Design review of the part built by this model. Coordinates are the model's own, in mm. Face numbers are marked on the shaded views. A direction names the side the tool comes from. Give positions to 0.01 mm unless a question says otherwise; leave off trailing zeros. Loops run counter-clockwise (first coordinate to the right, second up) from the corner with the lowest first, then second, coordinate; pieces in that order, holes last. Notation, with made-up numbers: (75, -33) - (103, -33) arc R25 cw to (103, -7) - close; hole circle Ø3 at (36, -5). An arc over 180 degrees is marked (long way). Put each result on its own line as item: value. Start each with the question number.
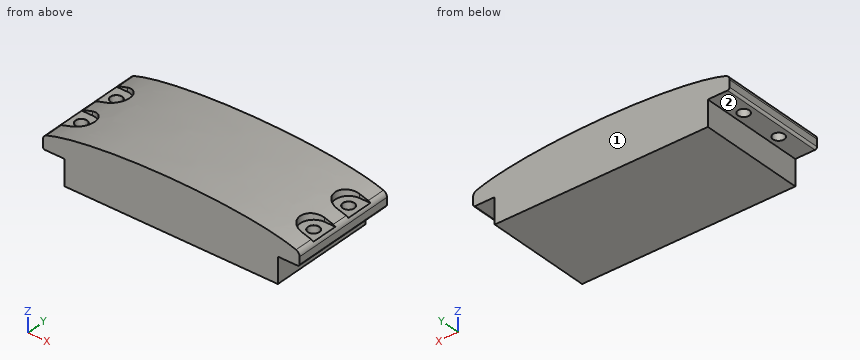
```python
from build123d import *

# Parameters (mm, degrees)
BOSS_EXTRUDE1_DEPTH            = 31.75
SKETCH3_W                      = 3.6195
SKETCH3_H                      = 8
CUT_EXTRUDE1_DEPTH             = 51.990302463
M3_CLEARANCE_HOLE1_D           = 3.4
M3_CLEARANCE_HOLE1_CSINK_D     = 3.45
M3_CLEARANCE_HOLE1_CSINK_ANGLE = 100


with BuildPart() as part:
    # Sketch1 → Boss-Extrude1 (new body)
    with BuildSketch(Plane(origin=(0, 0, 0), x_dir=(1, 0, 0), z_dir=(0, 1, 0))):
        with BuildLine():
            Line((31.75, -7.62), (31.75, 0))
            Line((31.75, 0), (-31.75, 0))
            Line((-31.75, 0), (-31.75, -7.62))
            Line((-31.75, -7.62), (-37.465, -7.62))
            Line((-37.465, -7.62), (-37.592, -7.62))
            ThreePointArc((-37.592, -7.62), (-38.041012806, -7.805987194), (-38.227, -8.255))
            Line((-38.227, -8.255), (-38.227, -10.33620332))
            ThreePointArc((-38.227, -10.33620332), (-37.934339966, -11.254650768), (-37.164265243, -11.834461539))
            add(Edge.make_bspline(
                [(-37.164265243, -11.834461539), (0, -24.85125292), (37.164265243, -11.834461539)],
                knots=[0.466080532, 0.466080532, 0.466080532, 2.675512121, 2.675512121, 2.675512121], degree=2, weights=[0.959649984, 0.417495947, 0.959649984]))
            ThreePointArc((37.164265243, -11.834461539), (37.934339966, -11.254650768), (38.227, -10.33620332))
            Line((38.227, -10.33620332), (38.227, -8.255))
            ThreePointArc((38.227, -8.255), (38.041012806, -7.805987194), (37.592, -7.62))
            Line((37.592, -7.62), (37.465, -7.62))
            Line((37.465, -7.62), (31.75, -7.62))
        make_face()
    extrude(amount=BOSS_EXTRUDE1_DEPTH)

    # Sketch3 → Cut-Extrude1 (cut, through all)
    with BuildSketch(Plane.XY.offset(11.43)):
        with Locations((-36.41725, 22.225)):
            Rectangle(SKETCH3_W, SKETCH3_H)
        with BuildLine():
            ThreePointArc((-34.6075, 26.225), (-30.6075, 22.225), (-34.6075, 18.225))
            Line((-34.6075, 18.225), (-34.6075, 26.225))
        make_face()
        with Locations((-36.41725, 9.525)):
            Rectangle(SKETCH3_W, SKETCH3_H)
        with BuildLine():
            ThreePointArc((-34.6075, 13.525), (-30.6075, 9.525), (-34.6075, 5.525))
            Line((-34.6075, 5.525), (-34.6075, 13.525))
        make_face()
        with Locations((36.41725, 9.525)):
            Rectangle(SKETCH3_W, SKETCH3_H)
        with BuildLine():
            Line((34.6075, 13.525), (34.6075, 5.525))
            ThreePointArc((34.6075, 5.525), (30.6075, 9.525), (34.6075, 13.525))
        make_face()
        with Locations((36.41725, 22.225)):
            Rectangle(SKETCH3_W, SKETCH3_H)
        with BuildLine():
            Line((34.6075, 26.225), (34.6075, 18.225))
            ThreePointArc((34.6075, 18.225), (30.6075, 22.225), (34.6075, 26.225))
        make_face()
    extrude(amount=CUT_EXTRUDE1_DEPTH, mode=Mode.SUBTRACT)

    # M3 Clearance Hole1 (through all)
    with Locations(Plane.XY.offset(11.43)):
        with Locations((-34.6075, 22.225), (-34.6075, 9.525), (34.6075, 22.225), (34.6075, 9.525)):
            CounterSinkHole(M3_CLEARANCE_HOLE1_D / 2, M3_CLEARANCE_HOLE1_CSINK_D / 2, counter_sink_angle=M3_CLEARANCE_HOLE1_CSINK_ANGLE)


solid = part.part
```
Item 1: For P1, Ø8, axis at x = 35, y = 8.5, coming from the +Z side; P2, Ø2, axis at x = 32.5, y = 21, coming from the +Z side; P3, Ø4, axis at x = -14, y = 18, coming from the +Z side, all flat-tipped, find the tip position at first contact; note any pin that passes through.
Item 2: For L1, parallel to X at y = 23, z = 11; L2, parallel to Z at x = -1, y = 4.5; L3, parallel to X at y = 21, z = 8.75, list the stretches that pass through material, from the lowest coordinate up. Write a range as from..to.
Item 3: Consider section A-A (z = 3). State the section outline as (x, y) points.
Item 4: Machinability: for the marked faces 1 and 2, which of the approach directions +Z, -Z, +X, -X, +Y, -Y give a long, thin tool a straight path to every point of the face, cutting with its end or side? Answer none if there is none.
Geometry says:
1. P1: stops at z = 13.39
1. P2: stops at z = 11.43
1. P3: stops at z = 15.48
2. L1: x = -38.08..-36.12, -33.09..33.09, 36.12..38.08
2. L2: z = 0..15.78
2. L3: x = -38.23..-35.79, -33.43..33.43, 35.79..38.23
3. outline: (-31.75, 0) - (31.75, 0) - (31.75, 31.75) - (-31.75, 31.75) - close
4. face 1: +Z, -Z, +X, -X, +Y
4. face 2: -Z, -X, +Y, -Y
